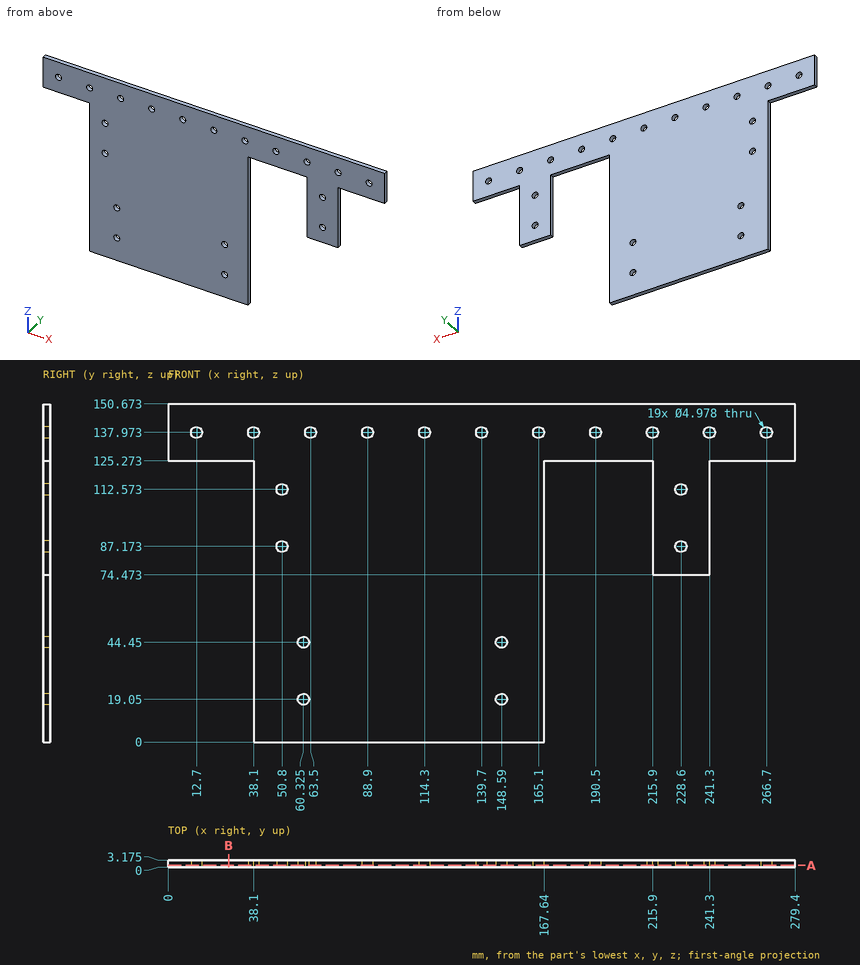
Part print with two shaded views. Sizes in mm from the minimum x, y, z corner. Coordinates: 2 decimals unless noted, no trailing zeros. Order: outer loops, then holes, each group sorted by start corner. A loop starts at its lowest first (then second) coordinate and runs counter-clockwise, first axis right, second up.
(1) Drill centre lines: L1, parallel to Z at x = 228.6, y = 1.55; L2, parallel to Z at x = 165.1, y = 0.7; L3, parallel to X at y = 0.2, z = 76.5. Where is each one in solid material? Low to high.
Solution:
L1: z = 74.47 to 84.68, 89.66 to 110.08, 115.06 to 150.67
L2: z = 0 to 135.48, 140.46 to 150.67
L3: x = 38.1 to 167.64, 215.9 to 241.3
(2) Pin check, flat tips, straight feed: pin 1 Ø8 at (x, z) = (50.8, 112.57) entering from -Y; pin 2 Ø3 at (x, z) = (228.6, 112.57) entering from -Y; pin 3 Ø1.6 at (x, y) = (183, 1.5) entering from -Z; pin 4 Ø1.6 at (x, y) = (230, 1.5) entering from -Z. Stop position of each tip, or through.
Solution:
pin 1: stops at y = 0
pin 2: passes through
pin 3: stops at z = 125.27
pin 4: stops at z = 74.47
(3) Saw through at B-B, the plane x = 27. Write the cut outline in (y, z) (1 decimal).
Solution:
outline: (0, 125.3) - (3.2, 125.3) - (3.2, 150.7) - (0, 150.7) - close
(4) Saw through at A-A, the plane y = 0.8. Count the separate pieces of the cut face and the enclosed holes in it, and give its area (3 significant figures).
Solution:
separate pieces: 1
enclosed holes: 19
area: 24,200 mm2
